Answer from the drawing. Dimensions are ordinates in mm from the lowest x, y and z of the part. A direction names the side the tool comes from. Give positions to 0.01 mm unless a question says otherwise; leave off trailing zeros. Order: outer loops, then holes, each group sorted by start corner. A loop starts at its lowest first (then second) coordinate and runs counter-clockwise, first axis right, second up. Notation, with made-up numbers: (61, -15) - (115, -15) arc R17 cw to (115, -9) - close; hole circle Ø10 at (85.5, 83). An arc over 180 degrees is marked (long way). Answer in a Markdown table with one row per item.
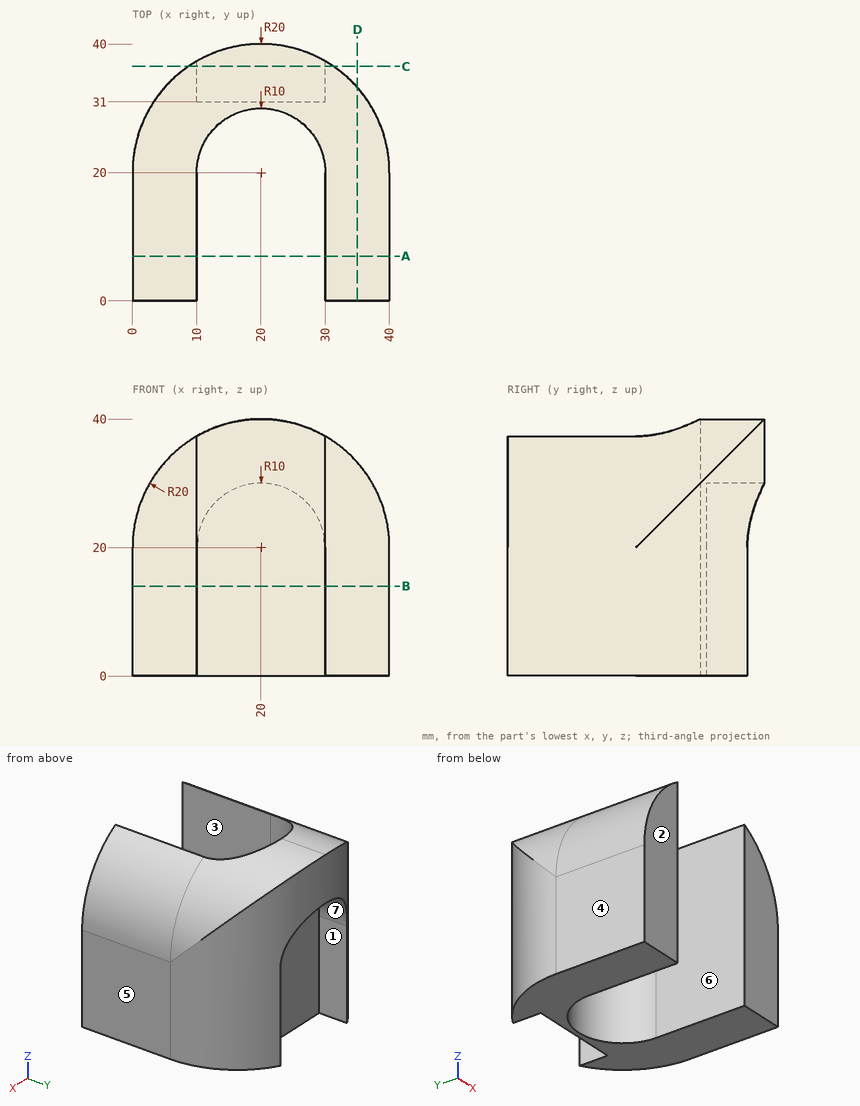
Item 1: Determine the mould class of the marked faces 1, 2, 3 and 4 for opening direction X: pulls with the +X half, pulls with the -X half, needs draft (parallel to the pull), parting line crosses it, or undercut.
Answer block:
| item | result |
|---|---|
| face 1 | undercut |
| face 2 | needs draft |
| face 3 | undercut |
| face 4 | pulls with the -X half |
Item 2: Which of the six approach directions +Z, -Z, +X, -X, +Y, -Y give full straight-line access (tool end or side, diameter ignored) to the marked faces 5, 6 and 7?
Answer block:
| item | result |
|---|---|
| face 5 | +Z, -Z, +X, +Y, -Y |
| face 6 | +Z, -Z, -Y |
| face 7 | -Z, +Y |
Item 3: Consider line 1 (X direction, y = 5, z = 15); line 2 (X direction, y = 24.5, z = 23); line 3 (Y direction, x = 20, z = 10). Determine where each line is inside the solid, lowest interval first.
Answer block:
| item | result |
|---|---|
| line 1 | 0 to 10, 30 to 40 |
| line 2 | 0.51 to 11.07, 28.93 to 39.49 |
| line 3 | 30 to 31 |
Item 4: Find section C-C on y = 36.5. Write down the section's boundary in (x, z), then the cut area to 3 significant figures.
Answer block:
| item | result |
|---|---|
| outline | (8.7, 0) - (10, 0) - (10, 20) arc R10 cw to (30, 20) - (30, 0) - (31.3, 0) - (31.3, 36.5) arc R20 ccw to (8.7, 36.5) - close |
| area | 322 mm² |
Item 5: Each of these flat-tipped pins is pushed along its axis until it touches: P1, Ø2, axis at x = 5, y = 20, coming from the +Z side; P2, Ø16, axis at x = 24.5, z = 16, coming from the +Y side; P3, Ø5, axis at y = 33.5, z = 15, coming from the +X side. Where does it stop, or does it pass through?
Answer block:
| item | result |
|---|---|
| P1 | z = 34.28 |
| P2 | y = 37.43 |
| P3 | x = 36.7 |
Item 6: Find section B-B on z = 14. Write down the section's boundary in (x, y), then the cut area to 3 significant figures.
Answer block:
| item | result |
|---|---|
| outline | (0, 0) - (10, 0) - (10, 20) arc R10 cw to (30, 20) - (30, 0) - (40, 0) - (40, 20) arc R20 ccw to (30, 37.32) - (30, 31) - (10, 31) - (10, 37.32) arc R20 ccw to (0, 20) - close |
| area | 709 mm² |
Item 7: Find section A-A on y = 7. Write down the section's boundary in (x, z).
Answer block:
| item | result |
|---|---|
| outline | (0, 0) - (10, 0) - (10, 37.32) arc R20 ccw to (0, 20) - close; (30, 0) - (40, 0) - (40, 20) arc R20 ccw to (30, 37.32) - close |
Item 8: Find section D-D on x = 35. Write down the section's boundary in (y, z).
Answer block:
| item | result |
|---|---|
| outline | (0, 0) - (33.23, 0) - (33.23, 33.23) - (0, 33.23) - close |
